Part print with two shaded views. Sizes in mm from the minimum x, y, z corner. A direction names the side the tool comes from. Round coordinates to 2 decimals unless told otherwise and drop trailing zeros. Loops run counter-clockwise (first coordinate to the right, second up) from the corner with the lowest first, then second, coordinate; pieces in that order, holes last.
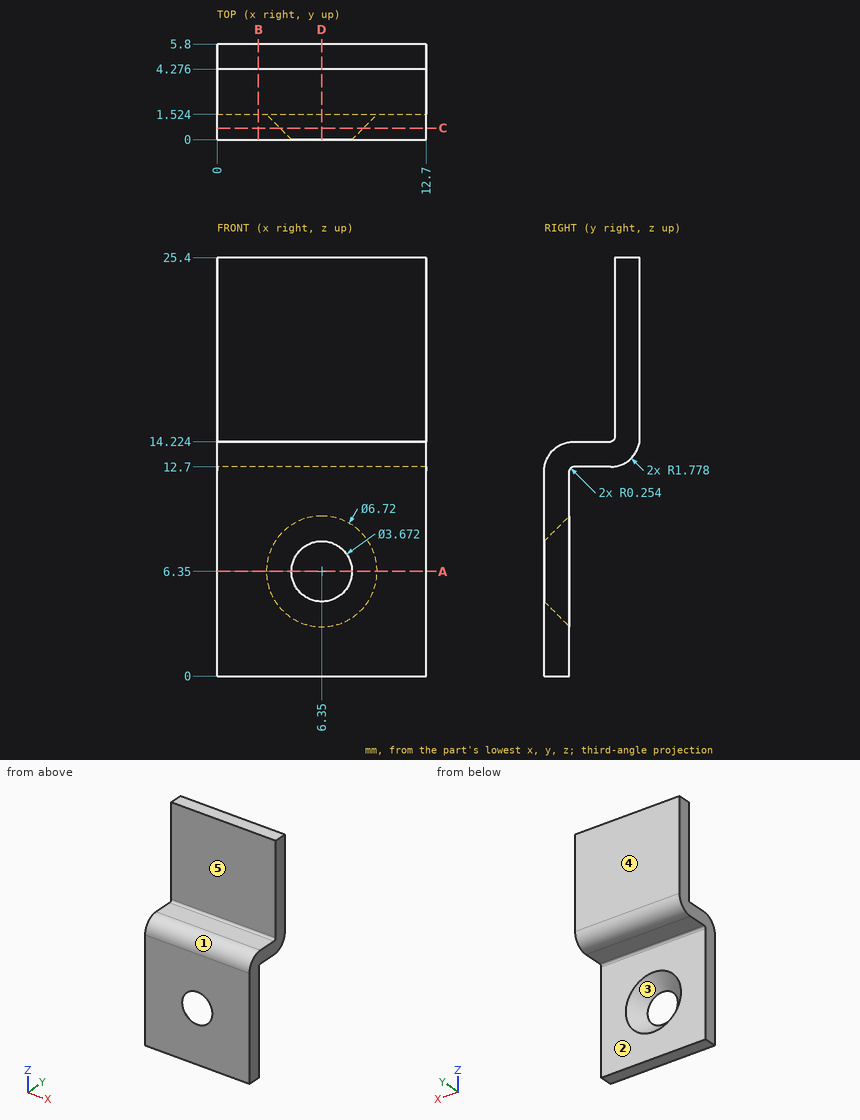
Item 1: Cut at A-A (z = 6.35). List the corners of the cut face in (x, y), plus the area to 3 significant figures.
Verdict:
outline: (0, 0) - (4.51, 0) - (2.99, 1.52) - (0, 1.52) - close; (8.19, 0) - (12.7, 0) - (12.7, 1.52) - (9.71, 1.52) - close
area: 11.4 mm2
Item 2: Cut at C-C (y = 0.7). List the corners of the cut face in (x, z).
Verdict:
outline: (0, 0) - (12.7, 0) - (12.7, 13.86) - (0, 13.86) - close; hole circle Ø5.07 at (6.35, 6.35)
Item 3: Mould opens along Z. For the marked faces 1, 2 and 3 say: released by +Z, released by -Z, zero draft, split by the parting line, or undercut.
Verdict:
face 1: released by +Z
face 2: zero draft
face 3: undercut
Item 4: Cut at D-D (x = 6.35). List the corners of the cut face in (y, z).
Verdict:
outline: (0, 0) - (1.52, 0) - (1.52, 2.99) - (0, 4.51) - close; (0, 8.19) - (1.52, 9.71) - (1.52, 12.45) arc R0.25 cw to (1.78, 12.7) - (4.02, 12.7) arc R1.78 ccw to (5.8, 14.48) - (5.8, 25.4) - (4.28, 25.4) - (4.28, 14.48) arc R0.25 cw to (4.02, 14.22) - (1.78, 14.22) arc R1.78 ccw to (0, 12.45) - close
Item 5: Flat gauge pins, fed straight in: P1, Ø1, axis at x = 3, y = 4, coming from the -Z side; P2, Ø3, axis at y = 4, z = 8, coming from the -X side; P3, Ø3.5, axis at x = 9, z = 3, coming from the +Y side; P4, Ø0.7, axis at x = 4.5, y = 3, coming from the +Z side. Where does each tip first touch, or does it go through?
Verdict:
P1: stops at z = 12.7
P2: passes through
P3: stops at y = 1.52
P4: stops at z = 14.22
Item 6: Wall check: L1, parallel to Z at x = 6, y = 2.2; L2, parallel to Y at x = 2.75, z = 23; L3, parallel to Z at x = 5, y = 0.75. Give the ranges that are in metal, low to high.
Verdict:
L1: z = 12.7 to 14.22
L2: y = 4.28 to 5.8
L3: z = 0 to 4.14, 8.56 to 13.9
Item 7: 3-axis set-ups, long thin cutter, end or side, ignore diameter. For the marked faces 4 and 5: which of +Z, -Z, +X, -X, +Y, -Y reach the whole face in a straight line?
Verdict:
face 4: +Z, -Z, +X, -X, +Y
face 5: +Z, +X, -X, -Y
Item 8: Cut at B-B (x = 2.5). List the corners of the cut face in (y, z).
Verdict:
outline: (0, 0) - (1.52, 0) - (1.52, 12.45) arc R0.25 cw to (1.78, 12.7) - (4.02, 12.7) arc R1.78 ccw to (5.8, 14.48) - (5.8, 25.4) - (4.28, 25.4) - (4.28, 14.48) arc R0.25 cw to (4.02, 14.22) - (1.78, 14.22) arc R1.78 ccw to (0, 12.45) - close
